from build123d import *

# Parameters (mm, degrees)
SKETCH_1_W          = 28
SKETCH_1_H          = 24
SKETCH_1_W_2        = 24
SKETCH_1_H_2        = 20
EXTRUDE_1_DEPTH     = 16
SKETCH_2_W          = 32
SKETCH_2_H          = 32
SKETCH_2_R          = 1.15
SKETCH_2_W_2        = 28
SKETCH_2_H_2        = 24
EXTRUDE_2_DEPTH     = 3
SKETCH_3_W          = 28
SKETCH_3_H          = 24
SKETCH_3_R          = 7.25
EXTRUDE_3_DEPTH     = 2
SKETCH_4_R          = 9.5
EXTRUDE_4_DEPTH     = 8
EXTRUDE_4_TAPER     = 3
SKETCH_6_R          = 7.25
CUT_EXTRUDE_2_DEPTH = 29.91366459
EXTRUDE_START       = -2
SKETCH_5_R          = 7.25
SKETCH_5_R_2        = 4.9
EXTRUDE_5_DEPTH     = 2
SKETCH_9_R          = 5.4
CUT_EXTRUDE_5_DEPTH = 1
FILLET_1_R          = 2
CUT_EXTRUDE_3_REACH = 36.467
SKETCH_7_W          = 20
SKETCH_7_H          = 5
CHAMFER_1_SIZE      = 2
SKETCH_8_R          = 2.25
CUT_EXTRUDE_4_DEPTH = 10
EXTRUDE_6_DEPTH     = 3
FILLET_2_R          = 2


with BuildPart() as part:
    # 草图1 → 凸台-拉伸1 (new body)
    with BuildSketch(Plane.XY):
        Rectangle(SKETCH_1_W, SKETCH_1_H)
        Rectangle(SKETCH_1_W_2, SKETCH_1_H_2, mode=Mode.SUBTRACT)
    extrude(amount=EXTRUDE_1_DEPTH)

    # 草图2 → 凸台-拉伸2 (add)
    with BuildSketch(Plane(origin=(0, 0, 0), x_dir=(-1, 0, 0), z_dir=(0, 0, -1))):
        Rectangle(SKETCH_2_W, SKETCH_2_H)
        with Locations((14, 14)):
            Circle(SKETCH_2_R, mode=Mode.SUBTRACT)
        with Locations((14, -14)):
            Circle(SKETCH_2_R, mode=Mode.SUBTRACT)
        with Locations((-14, -14)):
            Circle(SKETCH_2_R, mode=Mode.SUBTRACT)
        with Locations((-14, 14)):
            Circle(SKETCH_2_R, mode=Mode.SUBTRACT)
        Rectangle(SKETCH_2_W_2, SKETCH_2_H_2, mode=Mode.SUBTRACT)
    extrude(amount=-EXTRUDE_2_DEPTH)

    # 草图3 → 凸台-拉伸3 (add)
    with BuildSketch(Plane.XY.offset(16)):
        Rectangle(SKETCH_3_W, SKETCH_3_H)
        Circle(SKETCH_3_R, mode=Mode.SUBTRACT)
    extrude(amount=EXTRUDE_3_DEPTH)

    # 草图4 → 凸台-拉伸4 (add)
    with BuildSketch(Plane.XY.offset(18)):
        Circle(SKETCH_4_R)
    extrude(amount=EXTRUDE_4_DEPTH, taper=EXTRUDE_4_TAPER)

    # 草图6 → 切除-拉伸2 (cut, through all)
    with BuildSketch(Plane(origin=(0, 0, 18), x_dir=(-1, 0, 0), z_dir=(0, 0, -1))):
        Circle(SKETCH_6_R)
    extrude(amount=-CUT_EXTRUDE_2_DEPTH, mode=Mode.SUBTRACT)

    # 草图5 → 凸台-拉伸5 (add)
    with BuildSketch(Plane.XY.offset(26).offset(EXTRUDE_START)):
        Circle(SKETCH_5_R)
        Circle(SKETCH_5_R_2, mode=Mode.SUBTRACT)
    extrude(amount=EXTRUDE_5_DEPTH)

    # 草图9 → 切除-拉伸5 (cut)
    with BuildSketch(Plane.XY.offset(26)):
        Circle(SKETCH_9_R)
    extrude(amount=-CUT_EXTRUDE_5_DEPTH, mode=Mode.SUBTRACT)

    # 圆角1
    fillet_1_edges = [part.edges().sort_by_distance(p)[0] for p in [
        (12, -10, 8),
        (12, 10, 8),
        (-12, 10, 8),
        (-12, -10, 8),
        (14, -12, 10.5),
        (-14, -12, 10.5),
        (-14, 12, 10.5),
        (14, 12, 10.5),
    ]]
    fillet(fillet_1_edges, radius=FILLET_1_R)

    # 草图7 → 切除-拉伸3 (cut, up to next)
    with BuildSketch(Plane(origin=(0, 0, 0), x_dir=(-1, 0, 0), z_dir=(0, 0, -1)), mode=Mode.PRIVATE) as cut_extrude_3_sk1:
        with Locations((0, 14.7)):
            Rectangle(SKETCH_7_W, SKETCH_7_H)
    cut_extrude_3_tool1 = extrude(cut_extrude_3_sk1.sketch, amount=-CUT_EXTRUDE_3_REACH, mode=Mode.PRIVATE) & part.part
    add(cut_extrude_3_tool1.solids().sort_by_distance((0, 14.7, 0))[0], mode=Mode.SUBTRACT)

    # 倒角1
    # the kernel refuses this chamfer: 2 mm, written as the material it adds along each edge
    with BuildSketch(Plane(origin=(-12, 12, 3), x_dir=(0, 1, 0), z_dir=(1, 0, 0))) as chamfer_1_piece_1_section:
        Polygon((CHAMFER_1_SIZE, 0), (0, CHAMFER_1_SIZE), (0, 0), align=None)
    chamfer_1_piece_1 = extrude(amount=24, mode=Mode.PRIVATE)
    chamfer_1_piece_1 = split(chamfer_1_piece_1, bisect_by=Plane(origin=(-12, 12.2, 3), z_dir=(0, 1, 0)), keep=Keep.TOP, mode=Mode.PRIVATE)
    chamfer_1_piece_1 = split(chamfer_1_piece_1, bisect_by=Plane(origin=(-10, 12, 3), z_dir=(-1, 0, 0)), keep=Keep.TOP, mode=Mode.PRIVATE)
    add(chamfer_1_piece_1)
    with BuildSketch(Plane(origin=(-12, 12, 3), x_dir=(0, 1, 0), z_dir=(1, 0, 0))) as chamfer_1_piece_2_section:
        Polygon((CHAMFER_1_SIZE, 0), (0, CHAMFER_1_SIZE), (0, 0), align=None)
    chamfer_1_piece_2 = extrude(amount=24, mode=Mode.PRIVATE)
    chamfer_1_piece_2 = split(chamfer_1_piece_2, bisect_by=Plane(origin=(-12, 12.2, 3), z_dir=(0, -1, 0)), keep=Keep.TOP, mode=Mode.PRIVATE)
    chamfer_1_piece_2 = split(chamfer_1_piece_2, bisect_by=Plane(origin=(-10, 12, 3), z_dir=(-1, 0, 0)), keep=Keep.TOP, mode=Mode.PRIVATE)
    add(chamfer_1_piece_2)
    with BuildSketch(Plane(origin=(-12, 12, 3), x_dir=(0, 1, 0), z_dir=(1, 0, 0))) as chamfer_1_piece_3_section:
        Polygon((CHAMFER_1_SIZE, 0), (0, CHAMFER_1_SIZE), (0, 0), align=None)
    chamfer_1_piece_3 = extrude(amount=24, mode=Mode.PRIVATE)
    chamfer_1_piece_3 = split(chamfer_1_piece_3, bisect_by=Plane(origin=(10, 12, 3), z_dir=(-1, 0, 0)), keep=Keep.TOP, mode=Mode.PRIVATE)
    chamfer_1_piece_3 = split(chamfer_1_piece_3, bisect_by=Plane(origin=(-12, 12.2, 3), z_dir=(0, -1, 0)), keep=Keep.TOP, mode=Mode.PRIVATE)
    chamfer_1_piece_3 = split(chamfer_1_piece_3, bisect_by=Plane(origin=(-10, 12, 3), z_dir=(1, 0, 0)), keep=Keep.TOP, mode=Mode.PRIVATE)
    add(chamfer_1_piece_3)
    with BuildSketch(Plane(origin=(-12, 12, 3), x_dir=(0, 1, 0), z_dir=(1, 0, 0))) as chamfer_1_piece_4_section:
        Polygon((CHAMFER_1_SIZE, 0), (0, CHAMFER_1_SIZE), (0, 0), align=None)
    chamfer_1_piece_4 = extrude(amount=24, mode=Mode.PRIVATE)
    chamfer_1_piece_4 = split(chamfer_1_piece_4, bisect_by=Plane(origin=(10, 12, 3), z_dir=(1, 0, 0)), keep=Keep.TOP, mode=Mode.PRIVATE)
    chamfer_1_piece_4 = split(chamfer_1_piece_4, bisect_by=Plane(origin=(-12, 12.2, 3), z_dir=(0, 1, 0)), keep=Keep.TOP, mode=Mode.PRIVATE)
    add(chamfer_1_piece_4)
    with BuildSketch(Plane(origin=(-12, 12, 3), x_dir=(0, 1, 0), z_dir=(1, 0, 0))) as chamfer_1_piece_5_section:
        Polygon((CHAMFER_1_SIZE, 0), (0, CHAMFER_1_SIZE), (0, 0), align=None)
    chamfer_1_piece_5 = extrude(amount=24, mode=Mode.PRIVATE)
    chamfer_1_piece_5 = split(chamfer_1_piece_5, bisect_by=Plane(origin=(10, 12, 3), z_dir=(1, 0, 0)), keep=Keep.TOP, mode=Mode.PRIVATE)
    chamfer_1_piece_5 = split(chamfer_1_piece_5, bisect_by=Plane(origin=(-12, 12.2, 3), z_dir=(0, -1, 0)), keep=Keep.TOP, mode=Mode.PRIVATE)
    add(chamfer_1_piece_5)
    with BuildSketch(Plane(origin=(12, 10, 3), x_dir=(1, 0, 0), z_dir=(0, -1, 0))) as chamfer_1_piece_6_section:
        Polygon((2 + CHAMFER_1_SIZE, 0), (2, CHAMFER_1_SIZE), (2, 0), align=None)
    chamfer_1_piece_6 = revolve(axis=Axis((12, 10, 3), (0, 0, 1)), revolution_arc=90, mode=Mode.PRIVATE)
    chamfer_1_piece_6 = split(chamfer_1_piece_6, bisect_by=Plane(origin=(16, 10, 3), z_dir=(-1, 0, 0)), keep=Keep.TOP, mode=Mode.PRIVATE)
    chamfer_1_piece_6 = chamfer_1_piece_6 - Plane(origin=(14, 14, 3), x_dir=(-1, 0, 0), z_dir=(0, 0, -1)) * Cylinder(1.15, 16, mode=Mode.PRIVATE)
    add(chamfer_1_piece_6)
    with BuildSketch(Plane(origin=(-12, 10, 3), x_dir=(-1, 0, 0), z_dir=(0, -1, 0))) as chamfer_1_piece_7_section:
        Polygon((2 + CHAMFER_1_SIZE, 0), (2, -CHAMFER_1_SIZE), (2, 0), align=None)
    chamfer_1_piece_7 = revolve(axis=Axis((-12, 10, 3), (0, 0, -1)), revolution_arc=90, mode=Mode.PRIVATE)
    chamfer_1_piece_7 = split(chamfer_1_piece_7, bisect_by=Plane(origin=(-16, 10, 3), z_dir=(1, 0, 0)), keep=Keep.TOP, mode=Mode.PRIVATE)
    chamfer_1_piece_7 = chamfer_1_piece_7 - Plane(origin=(-14, 14, 3), x_dir=(-1, 0, 0), z_dir=(0, 0, -1)) * Cylinder(1.15, 17, mode=Mode.PRIVATE)
    add(chamfer_1_piece_7)
    with BuildSketch(Plane(origin=(14, 10, 3), x_dir=(1, 0, 0), z_dir=(0, -1, 0))) as chamfer_1_piece_8_section:
        Polygon((CHAMFER_1_SIZE, 0), (0, CHAMFER_1_SIZE), (0, 0), align=None)
    chamfer_1_piece_8 = extrude(amount=20, mode=Mode.PRIVATE)
    chamfer_1_piece_8 = split(chamfer_1_piece_8, bisect_by=Plane(origin=(16, 10, 3), z_dir=(-1, 0, 0)), keep=Keep.TOP, mode=Mode.PRIVATE)
    add(chamfer_1_piece_8)
    with BuildSketch(Plane(origin=(-14, -10, 3), x_dir=(-1, 0, 0), z_dir=(0, 1, 0))) as chamfer_1_piece_9_section:
        Polygon((CHAMFER_1_SIZE, 0), (0, CHAMFER_1_SIZE), (0, 0), align=None)
    chamfer_1_piece_9 = extrude(amount=20, mode=Mode.PRIVATE)
    chamfer_1_piece_9 = split(chamfer_1_piece_9, bisect_by=Plane(origin=(-16, -10, 3), z_dir=(1, 0, 0)), keep=Keep.TOP, mode=Mode.PRIVATE)
    add(chamfer_1_piece_9)
    with BuildSketch(Plane(origin=(12, -10, 3), x_dir=(0, -1, 0), z_dir=(-1, 0, 0))) as chamfer_1_piece_10_section:
        Polygon((2 + CHAMFER_1_SIZE, 0), (2, CHAMFER_1_SIZE), (2, 0), align=None)
    chamfer_1_piece_10 = revolve(axis=Axis((12, -10, 3), (0, 0, 1)), revolution_arc=90, mode=Mode.PRIVATE)
    chamfer_1_piece_10 = split(chamfer_1_piece_10, bisect_by=Plane(origin=(16, -10, 3), z_dir=(-1, 0, 0)), keep=Keep.TOP, mode=Mode.PRIVATE)
    chamfer_1_piece_10 = chamfer_1_piece_10 - Plane(origin=(14, -14, 3), x_dir=(-1, 0, 0), z_dir=(0, 0, -1)) * Cylinder(1.15, 16, mode=Mode.PRIVATE)
    add(chamfer_1_piece_10)
    with BuildSketch(Plane(origin=(-12, -10, 3), x_dir=(0, -1, 0), z_dir=(1, 0, 0))) as chamfer_1_piece_11_section:
        Polygon((2 + CHAMFER_1_SIZE, 0), (2, -CHAMFER_1_SIZE), (2, 0), align=None)
    chamfer_1_piece_11 = revolve(axis=Axis((-12, -10, 3), (0, 0, -1)), revolution_arc=90, mode=Mode.PRIVATE)
    chamfer_1_piece_11 = split(chamfer_1_piece_11, bisect_by=Plane(origin=(-16, -10, 3), z_dir=(1, 0, 0)), keep=Keep.TOP, mode=Mode.PRIVATE)
    chamfer_1_piece_11 = chamfer_1_piece_11 - Plane(origin=(-14, -14, 3), x_dir=(-1, 0, 0), z_dir=(0, 0, -1)) * Cylinder(1.15, 17, mode=Mode.PRIVATE)
    add(chamfer_1_piece_11)
    with BuildSketch(Plane(origin=(12, -12, 3), x_dir=(0, 0, 1), z_dir=(-1, 0, 0))) as chamfer_1_piece_12:
        Polygon((CHAMFER_1_SIZE, 0), (0, -CHAMFER_1_SIZE), (0, 0), align=None)
    extrude(amount=24)

    # 草图8 → 切除-拉伸4 (cut)
    with BuildSketch(Plane.XY.offset(3)):
        with Locations((-14, -14)):
            Circle(SKETCH_8_R)
        with Locations((14, -14)):
            Circle(SKETCH_8_R)
        with Locations((14, 14)):
            Circle(SKETCH_8_R)
        with Locations((-14, 14)):
            Circle(SKETCH_8_R)
    extrude(amount=CUT_EXTRUDE_4_DEPTH, mode=Mode.SUBTRACT)

    # 草图10 → 凸台-拉伸6 (add)
    with BuildSketch(Plane.XY.offset(3)):
        with BuildLine():
            Line((16, -16), (16, -11.127718677))
            ThreePointArc((16, -11.127718677), (16.474873734, -16.474873734), (11.127718677, -16))
            Line((11.127718677, -16), (16, -16))
        make_face()
        with BuildLine():
            Line((-16, -16), (-11.127718677, -16))
            ThreePointArc((-11.127718677, -16), (-16.474873734, -16.474873734), (-16, -11.127718677))
            Line((-16, -11.127718677), (-16, -16))
        make_face()
        with BuildLine():
            Line((-16, 16), (-11.127718677, 16))
            ThreePointArc((-11.127718677, 16), (-16.474873734, 16.474873734), (-16, 11.127718677))
            Line((-16, 11.127718677), (-16, 16))
        make_face()
        with BuildLine():
            Line((16, 16), (11.127718677, 16))
            ThreePointArc((11.127718677, 16), (16.474873734, 16.474873734), (16, 11.127718677))
            Line((16, 11.127718677), (16, 16))
        make_face()
    extrude(amount=-EXTRUDE_6_DEPTH)

    # 圆角2
    # the kernel refuses this fillet: 2 mm, written as the material it adds along each edge
    with BuildSketch(Plane(origin=(16, -11.127718677, 3), x_dir=(0, 1, 0), z_dir=(0, 0, -1)), Plane(origin=(-11.127718677, -16, 3), x_dir=(1, 0, 0), z_dir=(0, 0, -1)), Plane(origin=(-16, 11.127718677, 3), x_dir=(0, -1, 0), z_dir=(0, 0, -1))) as fillet_2_piece_1:
        with BuildLine():
            CenterArc((0.902635894, 2), FILLET_2_R, 226.658241773, 43.341758227)
            ThreePointArc((-0.470061276, 0.545454545), (-0.220966302, 0.284847622), (0, 0))
            Line((0, 0), (0.902635894, 0))
        make_face()
    extrude(amount=3)
    with BuildSketch(Plane(origin=(11.127718677, -16, 3), x_dir=(-1, 0, 0), z_dir=(0, 0, -1)), Plane(origin=(-16, -11.127718677, 3), x_dir=(0, 1, 0), z_dir=(0, 0, -1)), Plane(origin=(16, 11.127718677, 3), x_dir=(0, -1, 0), z_dir=(0, 0, -1))) as fillet_2_piece_2:
        with BuildLine():
            CenterArc((0.902635894, -2), FILLET_2_R, 90, 43.341758227)
            ThreePointArc((-0.470061276, -0.545454545), (-0.220966302, -0.284847622), (0, 0))
            Line((0, 0), (0.902635894, 0))
        make_face()
    extrude(amount=3)
    # the kernel refuses this fillet: 2 mm, written as the material it takes off along each edge
    with BuildSketch(Plane(origin=(-10, 16, 7.499392524), x_dir=(-1, 0, 0), z_dir=(0, 0, -1))) as fillet_2_2_piece_1:
        with BuildLine():
            CenterArc((2, -1.799757009), FILLET_2_R, 115.857898182, 64.142101818)
            Line((0, -1.799757009), (0, 0))
            Line((0, 0), (1.127718677, 0))
        make_face()
    extrude(amount=11.998785047, mode=Mode.SUBTRACT)
    with BuildSketch(Plane(origin=(10, 16, -4.499392524), x_dir=(0, -1, 0), z_dir=(0, 0, 1))) as fillet_2_2_piece_2:
        with BuildLine():
            CenterArc((1.799757009, 2), FILLET_2_R, 205.857898182, 64.142101818)
            Line((0, 1.127718677), (0, 0))
            Line((0, 0), (1.799757009, 0))
        make_face()
    extrude(amount=11.998785047, mode=Mode.SUBTRACT)


solid = part.part
Design review of the part built by this model. Coordinates are the model's own, in mm. A direction names the side the tool comes from. Coordinates: 2 decimals unless noted, no trailing zeros. Write each loop counter-clockwise with the first axis right and the second up, starting at its lowest first coordinate (ties: lowest second). Pieces come first, ordered by that corner, then holes. Notation, with made-up numbers: (-38.75, 0.25) - (17.25, 0.25) arc R30 ccw to (17.25, 39.25) - close; hole circle Ø3 at (58.25, -5.5). An arc over 180 degrees is marked (long way). Use one line per item in the form item = value.
Q1. Machinability: for faces 1 (the cylindrical face through (-11.43, -9.4, 8.11)), 2 (the flat face through (-16, 0, 1)), 3 (the flat face through (16, 0, 1)), which of the approach directions +Z, -Z, +X, -X, +Y, -Y give a long, thin tool a straight path to every point of the face, cutting with its end or side? Answer none if there is none.
Taken from the geometry:
face_1 = -Z
face_2 = +Z, -Z, -X
face_3 = +Z, -Z, +X
Q2. Consider section C-C (z = 12). Write out the cut boundary in (x, y), plus the area to 3 significant figures.
Taken from the geometry:
outline = (-14, -10) arc R2 ccw to (-12, -12) - (12, -12) arc R2 ccw to (14, -10) - (14, 10) arc R2 ccw to (12, 12) - (-12, 12) arc R2 ccw to (-14, 10) - close; hole (-12, -8) arc R2 ccw to (-10, -10) - (10, -10) arc R2 ccw to (12, -8) - (12, 8) arc R2 ccw to (10, 10) - (-10, 10) arc R2 ccw to (-12, 8) - close
area = 192 mm^2
Q3. For probe 1 along Y at (x, z) = (14, 1.6); probe 2 along Y at (x, z) = (6.5, 7.25); probe 3 along Z at (x, y) = (7.5, 3.5), list the stretches that pass through material, from the lowest coordinate up.
Taken from the geometry:
probe_1 = -17.5 to -15.15, -12.85 to 12.85, 15.15 to 17.5
probe_2 = -12 to -10, 10 to 12
probe_3 = 16 to 26
Q4. Consider section D-D (z = 1.75). Count the separate pieces of the cut face and the enclosed holes in it, plus the area to 3 significant figures.
Taken from the geometry:
separate_pieces = 1
enclosed_holes = 5
area = 501 mm^2
Q5. Consider section B-B (y = 0). Write out the cut boundary in (x, z), plus the area to 3 significant figures.
Taken from the geometry:
outline = (-16, 0) - (-12, 0) - (-12, 16) - (-7.25, 16) - (-7.25, 24) - (-4.9, 24) - (-4.9, 25) - (-5.4, 25) - (-5.4, 26) - (-9.08, 26) - (-9.5, 18) - (-14, 18) - (-14, 5) - (-16, 3) - close; (4.9, 24) - (7.25, 24) - (7.25, 16) - (12, 16) - (12, 0) - (16, 0) - (16, 3) - (14, 5) - (14, 18) - (9.5, 18) - (9.08, 26) - (5.4, 26) - (5.4, 25) - (4.9, 25) - close
area = 148 mm^2
Q6. The part is to be moulded in two halves that separate along Y. For faces 4 (the cylindrical face through (-12.959, -12.005, 3.679)), 5 (the cylindrical face through (-1.17, -5.27, 25.51)), 6 (the flat face through (-10, 0, 18)), say which applies: +Y half, -Y half, draft (parallel to the pull), parting line (faces both ways), or undercut.
Taken from the geometry:
face_4 = -Y half
face_5 = undercut
face_6 = draft
Q7. Insertion check: pin 1 Ø3.5 at (y, z) = (-4, 2) entering from -X; pin 2 Ø2 at (x, y) = (-13.5, 12) entering from +Z; pin 3 Ø3 at (x, y) = (-14, 14) entering from -Z; pin 4 Ø4 at (y, z) = (-3.5, 5.5) entering from +X. Each pin has a flat end and moves straight along its axis. Give the tip position at first contact, or say it passes through.
Taken from the geometry:
pin_1 = -16
pin_2 = 18
pin_3 = 0
pin_4 = 15.5
